The drawing under review shows one solid part. Ordinate dimensions are in mm from its lowest x, y, z. A direction names the side the tool comes from. Round coordinates to 2 decimals unless told otherwise and drop trailing zeros. Write each loop counter-clockwise with the first axis right and the second up, starting at its lowest first coordinate (ties: lowest second). Pieces come first, ordered by that corner, then holes. Notation, with made-up numbers: (-31.5, 81.5) - (14.5, 81.5) arc R22 cw to (14.5, 118.5) - close; hole circle Ø7 at (-29, 31). An arc over 180 degrees is marked (long way). Answer in a Markdown table with one row per item. Add a question column.
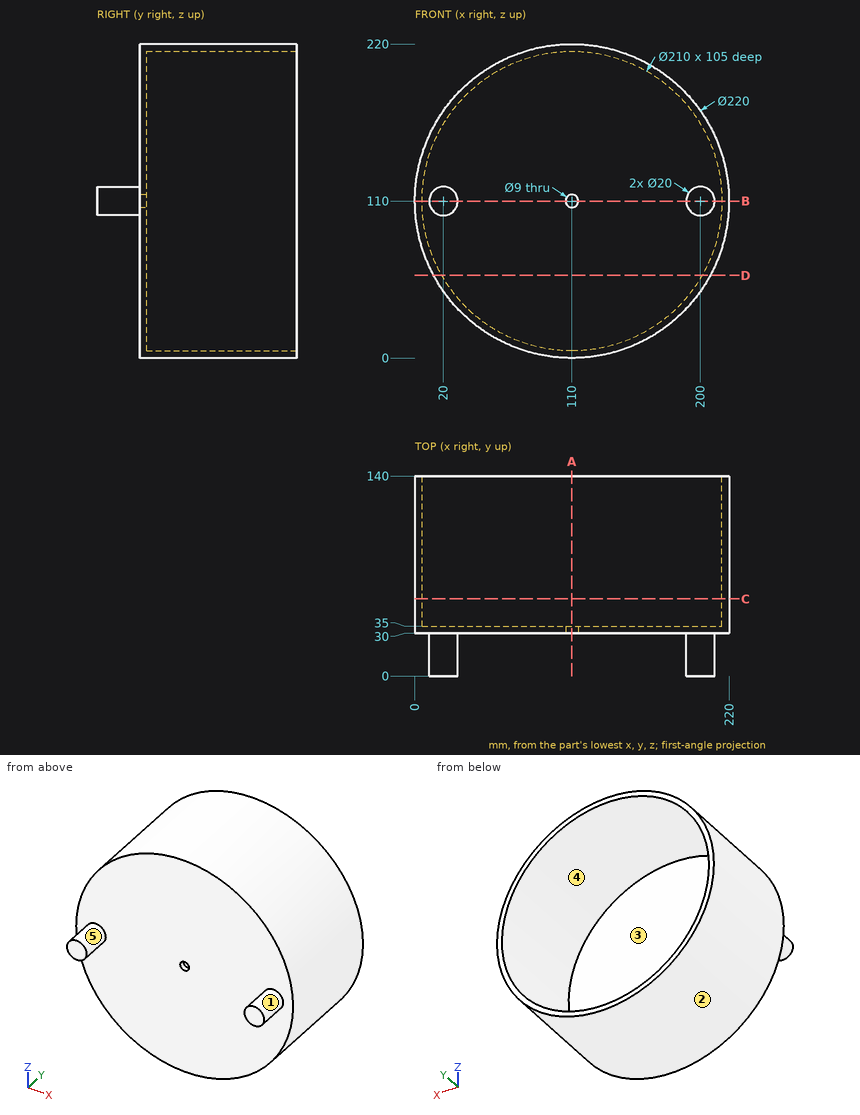
Q1. Draft analysis for pull direction X (two halves, no side actions). For the marked faces 1, 2 and 3, state which applies: released by +X, released by -X, zero draft, split by the parting line, or undercut.
Q2. Insertion check: pin 1 Ø1.5 at (y, z) = (116.5, 90) entering from +X; pin 2 Ø6 at (x, z) = (90, 158) entering from -Y; pin 3 Ø3 at (y, z) = (63.5, 123.5) entering from -X; pin 4 Ø12 at (x, y) = (128.5, 19) entering from -Z. Each pin has a flat end and moves straight along its axis. Give the tip position at first contact, or say it passes through.
Q3. Add section B-B on z = 110. State the section outline as (x, y) points.
Q4. Tool access review of the marked faces 4 and 5: name each direction out of +Z, -Z, +X, -X, +Y, -Y from which nothing blocks a thin tool from reaching the whole face with its end or side.
Q5. Add section A-A on x = 110. State the section outline as (y, z) points.
Q6. To check wall thickness, follow probe 1 along X at (y, z) = (68, 110); probe 2 along X at (y, z) = (33, 110); probe 3 along Z at (x, y) = (122, 64). State the ranges of each line that lie inside material, in increasing order.
Q7. Add section D-D on z = 58. State the section outline as (x, y) points, then the cut area to 3 significant figures.
Q8. Add section C-C on y = 54. State the section outline as (x, z) points.
Answer sheet:
| question | item | result |
|---|---|---|
| 1 | face 1 | undercut |
| 1 | face 2 | split by the parting line |
| 1 | face 3 | undercut |
| 2 | pin 1 | stops at x = 218.3 |
| 2 | pin 2 | stops at y = 30 |
| 2 | pin 3 | stops at x = 0.66 |
| 2 | pin 4 | passes through |
| 3 | outline | (0, 30) - (10, 30) - (10, 0) - (30, 0) - (30, 30) - (105.5, 30) - (105.5, 35) - (5, 35) - (5, 140) - (0, 140) - close; (114.5, 30) - (190, 30) - (190, 0) - (210, 0) - (210, 30) - (220, 30) - (220, 140) - (215, 140) - (215, 35) - (114.5, 35) - close |
| 4 | face 4 | +Y |
| 4 | face 5 | -Y |
| 5 | outline | (30, 0) - (140, 0) - (140, 5) - (35, 5) - (35, 105.5) - (30, 105.5) - close; (30, 114.5) - (35, 114.5) - (35, 215) - (140, 215) - (140, 220) - (30, 220) - close |
| 6 | probe 1 | x = 0 to 5, 215 to 220 |
| 6 | probe 2 | x = 0 to 105.5, 114.5 to 220 |
| 6 | probe 3 | z = 0.66 to 5.69, 214.31 to 219.34 |
| 7 | outline | (13.07, 30) - (206.93, 30) - (206.93, 140) - (201.22, 140) - (201.22, 35) - (18.78, 35) - (18.78, 140) - (13.07, 140) - close |
| 7 | area | 2,170 mm² |
| 8 | outline | circle Ø220 at (110, 110); hole circle Ø210 at (110, 110) |
